from build123d import *

# Parameters (mm, degrees)
CUT_EXTRUDE_1_DEPTH = 24.5
SKETCH_4_W          = 10
SKETCH_4_H          = 10.423116616
CUT_EXTRUDE_2_DEPTH = 111.376079444


with BuildPart() as part:
    # Эскиз1 → Повернуть1 (revolve)
    with BuildSketch(Plane.XY, mode=Mode.PRIVATE) as revolve_1_sk:
        with BuildLine():
            Line((-70.245087719, -6.642192982), (-69.245087719, -7.642192982))
            Line((-69.245087719, -7.642192982), (9.254912281, -7.642192982))
            Line((9.254912281, -7.642192982), (10.254912281, -6.642192982))
            Line((10.254912281, -6.642192982), (10.254912281, 23.357807018))
            Line((10.254912281, 23.357807018), (9.254912281, 24.357807018))
            Line((9.254912281, 24.357807018), (-20.745087719, 24.357807018))
            ThreePointArc((-20.745087719, 24.357807018), (-23.927068235, 23.039787533), (-25.245087719, 19.857807018))
            Line((-25.245087719, 19.857807018), (-25.245087719, 19.357807018))
            ThreePointArc((-25.245087719, 19.357807018), (-26.563107204, 16.175826502), (-29.745087719, 14.857807018))
            Line((-29.745087719, 14.857807018), (-65.745087719, 14.857807018))
            ThreePointArc((-65.745087719, 14.857807018), (-68.927068235, 13.539787533), (-70.245087719, 10.357807018))
            Line((-70.245087719, 10.357807018), (-70.245087719, -6.642192982))
        make_face()
    revolve(revolve_1_sk.sketch.rotate(Axis((-70.245087719, -27.642192982, 0), (1, 0, 0)), 90), axis=Axis((-70.245087719, -27.642192982, 0), (1, 0, 0)))

    # Эскиз3 → Вырез-Вытянуть1 (cut)
    with BuildSketch(Plane(origin=(10.254912281, 0, 0), x_dir=(0, 0, -1), z_dir=(1, 0, 0))):
        with BuildLine():
            ThreePointArc((-17.761912417, -53.049169727), (0, -95.642192982), (17.761912417, -53.049169727))
            ThreePointArc((17.761912417, -53.049169727), (21.920310217, -49.562503199), (25.406976744, -45.4041054))
            ThreePointArc((25.406976744, -45.4041054), (68, -27.642192982), (25.406976744, -9.880280565))
            ThreePointArc((25.406976744, -9.880280565), (21.920310217, -5.721882766), (17.761912417, -2.235216238))
            ThreePointArc((17.761912417, -2.235216238), (0, 40.357807018), (-17.761912417, -2.235216238))
            ThreePointArc((-17.761912417, -2.235216238), (-21.920310217, -5.721882766), (-25.406976744, -9.880280565))
            ThreePointArc((-25.406976744, -9.880280565), (-68, -27.642192982), (-25.406976744, -45.4041054))
            ThreePointArc((-25.406976744, -45.4041054), (-21.920310217, -49.562503199), (-17.761912417, -53.049169727))
        make_face()
    extrude(amount=-CUT_EXTRUDE_1_DEPTH, mode=Mode.SUBTRACT)

    # Эскиз4 → Вырез-Вытянуть2 (cut, through all)
    with BuildSketch(Plane(origin=(-14.245087719, 0, 0), x_dir=(0, 0, -1), z_dir=(1, 0, 0))):
        with Locations((0, -8.85375129)):
            Rectangle(SKETCH_4_W, SKETCH_4_H)
    extrude(amount=-CUT_EXTRUDE_2_DEPTH, mode=Mode.SUBTRACT)


solid = part.part
Build history of the part. All positions in model axes, mm. A direction names the side the tool comes from. Coordinates: 2 decimals unless noted, no trailing zeros. Order: outer loops, then holes, each group sorted by start corner. A loop starts at its lowest first (then second) coordinate and runs counter-clockwise, first axis right, second up. Notation, with made-up numbers: (-12, 80.5) -> (-6, 80.5) arc R10 cw to (-6, 95.5) -> close; hole circle Ø7 at (-12.75, -32.5). An arc over 180 degrees is marked (long way). One line per item, written item: value.
(1) Probe line 1 (Y direction, x = -36, z = 0); line 2 (Z direction, x = -20.5, y = -18); line 3 (Y direction, x = -26, z = -8). List the from-to ranges inside material, lowest first. Write a range as [from, to].
Checked values:
line 1: [-70.14, -47.64], [-3.64, 14.86]
line 2: [-51.1, -17.52], [17.52, 51.1]
line 3: [-71.42, -45.97], [-9.31, 16.14]
(2) Tool access for faces 1 (the flat face through (-42, -6, -5)), 2 (the flat face through (-70.245, -11, 16)), 3 (the cylindrical face through (-1.82, -51.29, 34.89)): list every direction of +Z, -Z, +X, -X, +Y, -Y with a clear straight run to the whole face (end or side of a thin tool).
Checked values:
face 1: +X, -X
face 2: +Z, -Z, -X, +Y, -Y
face 3: +X
(3) Slice it at B-B, the plane x = -1.5. List the corners of the cut face in (y, z), plus the area to 3 significant figures.
Checked values:
outline: (-73.32, -24.86) arc R52 ccw to (-52.5, -45.67) arc R25 cw to (-45.4, -25.41) arc R31 cw to (-53.05, -17.76) arc R25 cw to start; (-73.32, 24.86) arc R25 cw to (-53.05, 17.76) arc R31 cw to (-45.4, 25.41) arc R25 cw to (-52.5, 45.67) arc R52 ccw to start; (-9.88, -25.41) arc R25 cw to (-2.79, -45.67) arc R52 ccw to (18.03, -24.86) arc R25 cw to (-2.24, -17.76) arc R31 cw to start; (-9.88, 25.41) arc R31 cw to (-2.24, 17.76) arc R25 cw to (18.03, 24.86) arc R52 ccw to (-2.79, 45.67) arc R25 cw to start
area: 1,430 mm2
(4) Drop flat-ended pins along their axis: pin 1 Ø1.4 at (x, y) = (-34.5, -7) entering from -Z; pin 2 Ø1.5 at (x, y) = (-15, -65) entering from -Z; pin 3 Ø12 at (x, y) = (-21.5, 0) entering from +Z. Give the stop position or say it passes through.
Checked values:
pin 1: z = -37.53
pin 2: z = -36.93
pin 3: z = 47.27
(5) Slice it at A-A, the plane z = 0. List the corners of the cut face in (x, y).
Checked values:
outline: (-70.25, -65.64) arc R4.5 ccw to (-65.75, -70.14) -> (-29.75, -70.14) arc R4.5 cw to (-25.25, -74.64) -> (-25.25, -75.14) arc R4.5 ccw to (-20.75, -79.64) -> (-14.25, -79.64) -> (-14.25, -47.64) -> (-69.25, -47.64) -> (-70.25, -48.64) -> close; (-70.25, -3.64) -> (-14.25, -3.64) -> (-14.25, 24.36) -> (-20.75, 24.36) arc R4.5 ccw to (-25.25, 19.86) -> (-25.25, 19.36) arc R4.5 cw to (-29.75, 14.86) -> (-65.75, 14.86) arc R4.5 ccw to (-70.25, 10.36) -> close
(6) Slice it at C-C, the plane x = -51.5. List the corners of the cut face in (y, z), plus the area to 3 significant figures.
Checked values:
outline: circle Ø85 at (-27.64, 0); hole (-8.28, -5) -> (-3.64, -5) -> (-3.64, 5) -> (-8.28, 5) arc R20 ccw (long way) to start
area: 4,380 mm2
(7) Mould opens along Z. For faces 4 (the cylindrical face through (-1.8, -5.8, -22)), 5 (the conical face through (10.1, 8.4, -36.3)), 6 (the flat face through (10.255, 3, -31)) say: pulls with the +Z half, pulls with the -Z half, needs draft (parallel to the pull), parting line crosses it, or undercut.
Checked values:
face 4: undercut
face 5: pulls with the -Z half
face 6: needs draft
